Job drawing, mm, ordinate dimensions from the low corner. One solid piece. A direction names the side the tool comes from. Give positions to 0.01 mm unless a question says otherwise; leave off trailing zeros. Order: outer loops, then holes, each group sorted by start corner. A loop starts at its lowest first (then second) coordinate and runs counter-clockwise, first axis right, second up. Notation, with made-up numbers: (80, 18) - (117, 18) arc R26 cw to (117, 45) - close; hole circle Ø6 at (-25.75, -26.5). An arc over 180 degrees is marked (long way). Write each question's results on one line, items separated by ' | '. Start each with the question number.
1) Cut at D-D on x = 13. List the corners of the cut face in (y, z).
2) Cut at A-A on x = 38.5. List the corners of the cut face in (y, z).
3) Tool access for the marked faces 1, 2 and 3: list every direction of +Z, -Z, +X, -X, +Y, -Y with a clear straight run to the whole face (end or side of a thin tool).
4) Two-plate mould, pull along X, no slides. Class the marked faces 4, 5, 6 and 7: +X half, -X half, draft (parallel to the pull), parting line (faces both ways), or undercut.
5) Cut at B-B on z = 51.5. List the corners of the cut face in (x, y), plus the area to 3 significant figures.
6) Drop flat-ended pins along their axis: pin 1 Ø4 at (x, y) = (39.5, 3) entering from -Z; pin 2 Ø11.5 at (x, z) = (10, 80) entering from +Y; pin 3 Ø4 at (y, z) = (5, 5) entering from +X. Give the stop position or say it passes through.
7) Cut at C-C on y = 5. State how many separate pieces and enclosed holes the cut face has, plus the area to 3 significant figures.
8) Drill centre lines: line 1 along X through (y, z) = (6.25, 20); line 2 along X through (y, z) = (7.75, 64.5); line 3 along X through (y, z) = (5.75, 55.5). Where is each one in solid material? Low to high. Write a range as from..to.
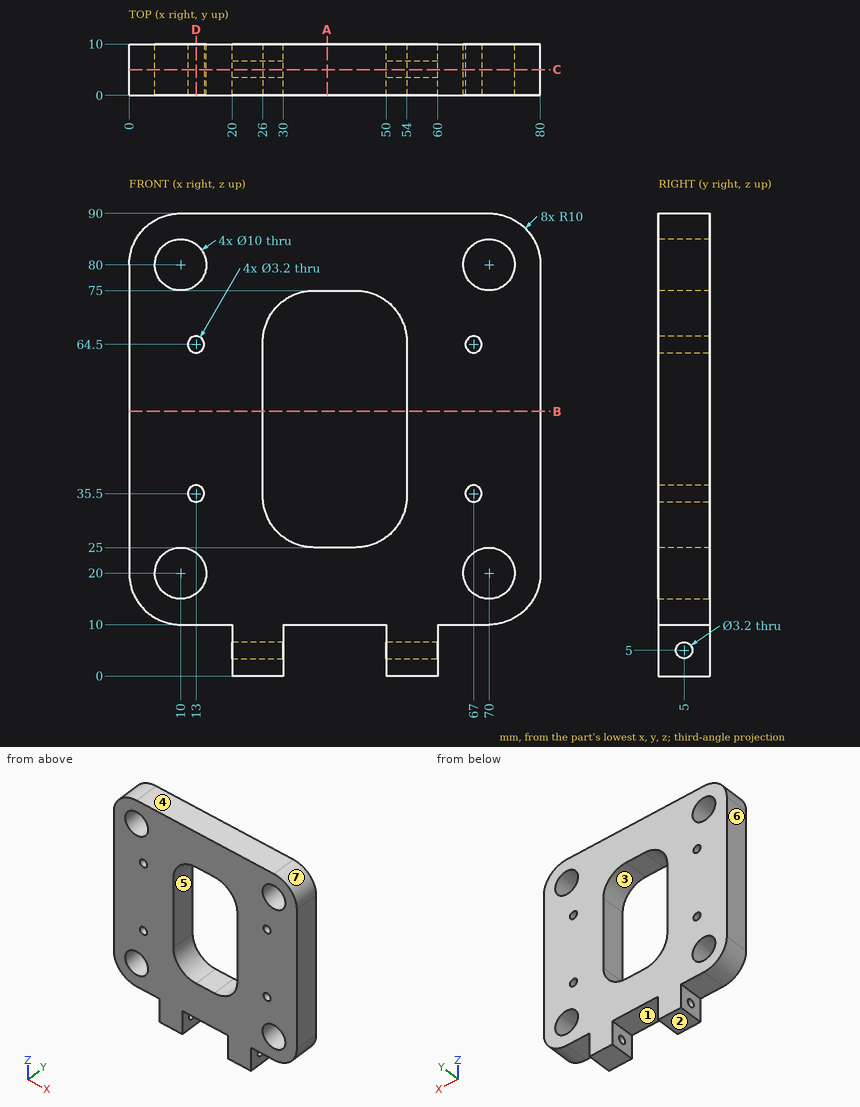
Results:
1) outline: (0, 10) - (10, 10) - (10, 16) - (0, 16) - close; (0, 24) - (10, 24) - (10, 33.9) - (0, 33.9) - close; (0, 37.1) - (10, 37.1) - (10, 62.9) - (0, 62.9) - close; (0, 66.1) - (10, 66.1) - (10, 76) - (0, 76) - close; (0, 84) - (10, 84) - (10, 90) - (0, 90) - close
2) outline: (0, 10) - (10, 10) - (10, 25) - (0, 25) - close; (0, 75) - (10, 75) - (10, 90) - (0, 90) - close
3) face 1: -Z, +Y, -Y | face 2: -Z, +X, -X, +Y, -Y | face 3: +Y, -Y
4) face 4: draft | face 5: undercut | face 6: -X half | face 7: +X half
5) outline: (0, 0) - (26, 0) - (26, 10) - (0, 10) - close; (54, 0) - (80, 0) - (80, 10) - (54, 10) - close | area: 520 mm^2
6) pin 1: z = 10 | pin 2: y = 10 | pin 3: x = 60
7) separate pieces: 3 | enclosed holes: 9 | area: 4,790 mm^2
8) line 1: 0..5, 15..65, 75..80 | line 2: 0..11.4, 14.6..26, 54..65.4, 68.6..80 | line 3: 0..26, 54..80
